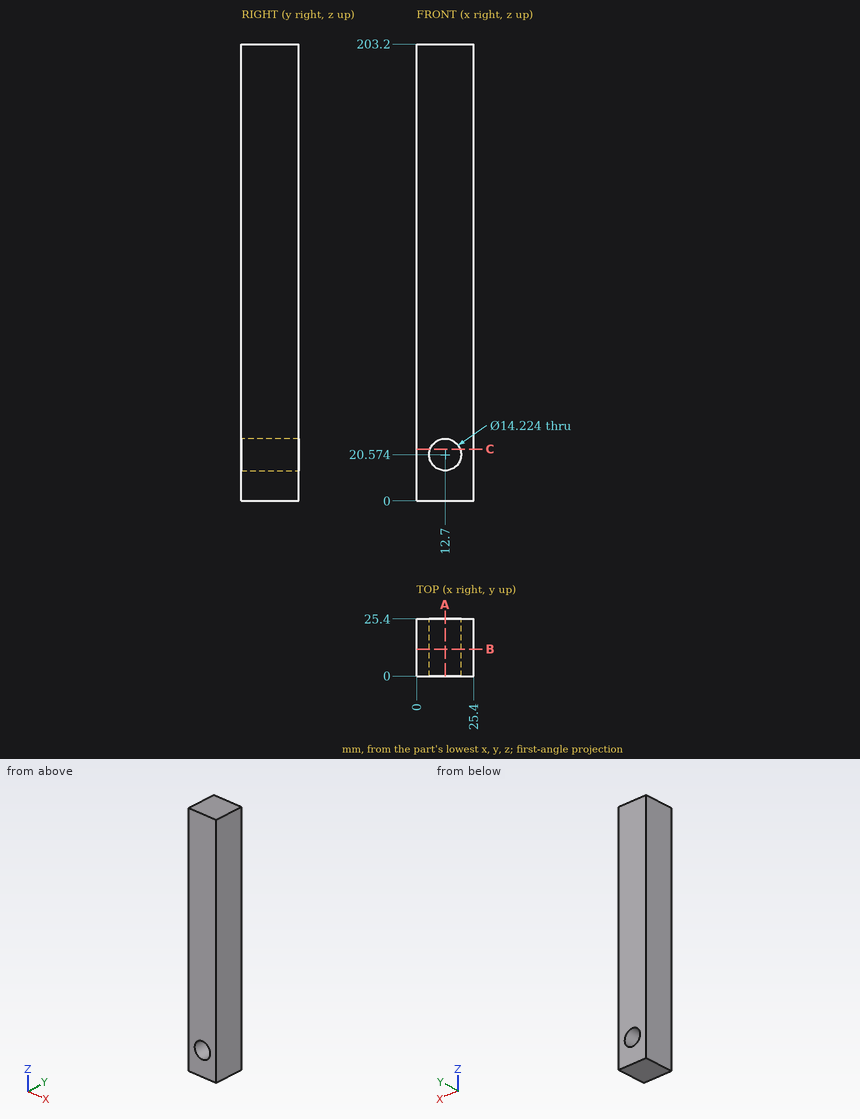
Study the drawing (mm; zero at the part's minimum x, y, z) and answer. Round coordinates to 2 decimals unless told otherwise and drop trailing zeros. Order: outer loops, then holes, each group sorted by start corner. A loop starts at its lowest first (then second) coordinate and runs counter-clockwise, first axis right, second up. Notation, with made-up numbers: (77, 85) - (114, 85) arc R33 ccw to (114, 116) - close; hole circle Ø6 at (8.5, -34.75). An arc over 180 degrees is marked (long way). Use one line per item in the form item = value. Start each with the question number.
(1) Find the intervals of material crossed by line 1 along Z through (x, y) = (12.75, 4); line 2 along Z through (x, y) = (11.5, 10.75), in increasing order. Write a range as from..to.
(2) The part is cut by section C-C (z = 23). Give the vertices of the cut face in (x, y), then the cut area to 3 significant figures.
(3) A flat-ended cylindrical pin translates along its axis: pin 1 Ø8.5 at (x, z) = (12.7, 20.574) entering from -Y. Find the tip coordinate at first contact, or state that the pin passes through.
(4) The part is cut by section A-A (x = 12.7). Give the vertices of the cut face in (y, z).
(5) The part is cut by section B-B (y = 12). Give the vertices of the cut face in (x, z).
Checked values:
q1.line_1 = 0..13.46, 27.69..203.2
q1.line_2 = 0..13.56, 27.58..203.2
q2.outline = (0, 0) - (6.01, 0) - (6.01, 25.4) - (0, 25.4) - close; (19.39, 0) - (25.4, 0) - (25.4, 25.4) - (19.39, 25.4) - close
q2.area = 306 mm^2
q3.pin_1 = through
q4.outline = (0, 0) - (25.4, 0) - (25.4, 13.46) - (0, 13.46) - close; (0, 27.69) - (25.4, 27.69) - (25.4, 203.2) - (0, 203.2) - close
q5.outline = (0, 0) - (25.4, 0) - (25.4, 203.2) - (0, 203.2) - close; hole circle Ø14.22 at (12.7, 20.57)
